The model under review builds one solid part; all positions refer to its coordinate system, in mm. Give positions to 0.01 mm unless a question says otherwise; leave off trailing zeros. Loops run counter-clockwise (first coordinate to the right, second up) from the corner with the lowest first, then second, coordinate; pieces in that order, holes last. Notation, with made-up numbers: (9.5, 41) -> (65.5, 41) arc R15 ccw to (65.5, 52) -> close; hole circle Ø11 at (42, 67). An arc over 180 degrees is marked (long way). Write each question's results on one line, items separated by ' | '. Start each with the question number.
Q1. We need section B-B (x = -32). Write out the cut boundary in (y, z) (3 decimals).
Q2. We need section A-A (z = 0.9). Write out the cut boundary in (x, y) (3 decimals).
Q3. Insertion check: pin 1 Ø1.6 at (y, z) = (-8.5, 2) entering from -X (3 decimals); pin 2 Ø1 at (x, z) = (39.5, 1) entering from +Y (3 decimals). Each pin has a flat end and moves straight along its axis. Give the tip position at first contact, or say it passes through.
Q4. We need section C-C (y = -10.5). Write out the cut boundary in (x, z) (3 decimals).
Q5. Wall thickness on L1, parallel to X at y = 2.5, z = 0.3 (3 decimals); L2, parallel to Y at x = 22, z = 2.8 (3 decimals): over which ranges is each line inside the solid? List them lowest first. Write a range as [from, to].
from build123d import *

# Parameters (mm, degrees)
ESQUISSE2_W             = 200
ESQUISSE2_H             = 80
BOSS_EXTRU_1_DEPTH      = 3.175
ESQUISSE3_W             = 35
ESQUISSE3_H             = 3.175
ENL_V_MAT_EXTRU_1_DEPTH = 4.175
ESQUISSE4_W             = 3.175
ESQUISSE4_H             = 35
ENL_V_MAT_EXTRU_2_DEPTH = 4.175


with BuildPart() as part:
    # Esquisse2 → Boss.-Extru.1 (new body)
    with BuildSketch(Plane.XY):
        Rectangle(ESQUISSE2_W, ESQUISSE2_H)
    extrude(amount=BOSS_EXTRU_1_DEPTH)

    # Esquisse3 → Enlèv. mat.-Extru.1 (cut, through all)
    with BuildSketch(Plane.XY.offset(3.175)):
        with Locations((35, 38.4125)):
            Rectangle(ESQUISSE3_W, ESQUISSE3_H)
        with Locations((-35, 38.4125)):
            Rectangle(ESQUISSE3_W, ESQUISSE3_H)
    extrude(amount=-ENL_V_MAT_EXTRU_1_DEPTH, mode=Mode.SUBTRACT)

    # Esquisse4 → Enlèv. mat.-Extru.2 (cut, through all)
    with BuildSketch(Plane.XY.offset(3.175)):
        with Locations((-98.4125, 0)):
            Rectangle(ESQUISSE4_W, ESQUISSE4_H)
    enl_v_mat_extru_2 = extrude(amount=-ENL_V_MAT_EXTRU_2_DEPTH, mode=Mode.SUBTRACT)

    # Symétrie1: Enlèv. mat.-Extru.2 across plane
    add(enl_v_mat_extru_2.mirror(Plane(origin=(0, 0, 0), x_dir=(0, 0, 1), z_dir=(1, 0, 0))), mode=Mode.SUBTRACT)


solid = part.part
Output:
1) outline: (-40, 0) -> (36.825, 0) -> (36.825, 3.175) -> (-40, 3.175) -> close
2) outline: (-100, -40) -> (100, -40) -> (100, -17.5) -> (96.825, -17.5) -> (96.825, 17.5) -> (100, 17.5) -> (100, 40) -> (52.5, 40) -> (52.5, 36.825) -> (17.5, 36.825) -> (17.5, 40) -> (-17.5, 40) -> (-17.5, 36.825) -> (-52.5, 36.825) -> (-52.5, 40) -> (-100, 40) -> (-100, 17.5) -> (-96.825, 17.5) -> (-96.825, -17.5) -> (-100, -17.5) -> close
3) pin 1: x = -96.825 | pin 2: y = 36.825
4) outline: (-96.825, 0) -> (96.825, 0) -> (96.825, 3.175) -> (-96.825, 3.175) -> close
5) L1: [-96.825, 96.825] | L2: [-40, 36.825]
